Geometry: final body of the model. Coordinates: model frame, mm. Face numbers are marked on the shaded views. A direction names the side the tool comes from. Round coordinates to 2 decimals unless told otherwise and drop trailing zeros. Order: outer loops, then holes, each group sorted by start corner. A loop starts at its lowest first (then second) coordinate and runs counter-clockwise, first axis right, second up. Notation, with made-up numbers: (9.25, -15.5) -> (63.25, -15.5) arc R21 cw to (63.25, 7.5) -> close; hole circle Ø2 at (49, 86). An arc over 180 degrees is marked (long way). Put each result on its own line as item: value.
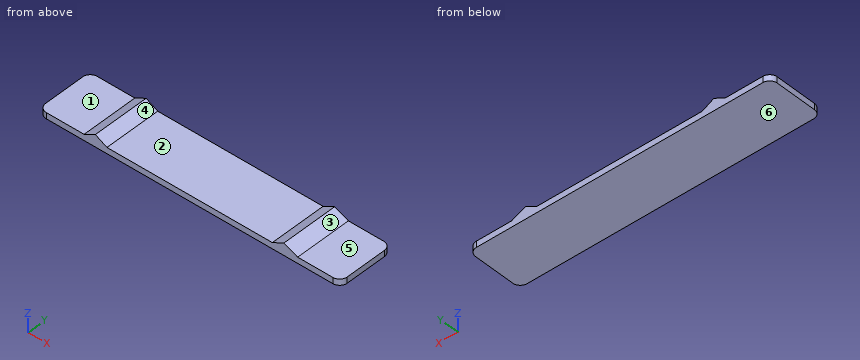
```python
from build123d import *

# Parameters (mm, degrees)
PAD_DEPTH = 7.5
FILLET_R  = 1


with BuildPart() as part:
    # Sketch → Pad (new body)
    with BuildSketch(Plane.XZ):
        Polygon((-20, -0.4), (20, -0.4), (20, 0.4), (14.320997, 0.4), (12.5, 1.2), (10.965424, 0.4), (-10.965424, 0.4), (-12.5, 1.2), (-13.994693, 0.4), (-20, 0.4), align=None)
    extrude(amount=PAD_DEPTH)

    # Fillet
    fillet_edges = [part.edges().sort_by_distance(p)[0] for p in [
        (-20, -7.5, 0),
        (-20, 0, 0),
        (20, 0, 0),
        (20, -7.5, 0),
    ]]
    fillet(fillet_edges, radius=FILLET_R)


solid = part.part
```
1. Draft query along X for the marked faces 1, 2 and 3. Return one class per face: +X half, -X half, draft (parallel to the pull), parting line (faces both ways), or undercut.
Ans:
face 1: draft
face 2: undercut
face 3: +X half
2. Cut plane D-D on y = -0.5. Return loops of the section in (x, z), and give its area (3 significant figures).
Ans:
outline: (-19.87, -0.4) -> (19.87, -0.4) -> (19.87, 0.4) -> (14.32, 0.4) -> (12.5, 1.2) -> (10.97, 0.4) -> (-10.97, 0.4) -> (-12.5, 1.2) -> (-13.99, 0.4) -> (-19.87, 0.4) -> close
area: 34.3 mm²
3. Contact query for a flat-ended pin moving along its axis: P1, Ø1.8, axis at x = -17, y = -5.5, coming from the +Z side. Output: stop coordinate, or through.
Ans:
P1: z = 0.4
4. Cut plane C-C on x = -0.5. Return loops of the section in (y, z).
Ans:
outline: (-7.5, -0.4) -> (0, -0.4) -> (0, 0.4) -> (-7.5, 0.4) -> close
5. Cut plane A-A on z = 0.85. Return loops of the section in (x, y).
Ans:
outline: (-13.15, -7.5) -> (-11.83, -7.5) -> (-11.83, 0) -> (-13.15, 0) -> close; (11.83, -7.5) -> (13.3, -7.5) -> (13.3, 0) -> (11.83, 0) -> close
6. Material intervals for probe 1 along Z at (x, y) = (-0.5, -1.25); probe 2 along X at (y, z) = (-3.5, 0.6); probe 3 along X at (y, z) = (-5, 0.5), sorted ascending.
Ans:
probe 1: -0.4 to 0.4
probe 2: -13.62 to -11.35, 11.35 to 13.87
probe 3: -13.81 to -11.16, 11.16 to 14.09
7. Set-up query: the marked faces 4, 5 and 6. Return all of +Z, -Z, +X, -X, +Y, -Y with unobstructed straight access to the full face (end or side cutting, diameter ignored); none if empty.
Ans:
face 4: +Z, +Y, -Y
face 5: +Z, +X, +Y, -Y
face 6: -Z, +X, -X, +Y, -Y
8. Cut plane B-B on y = -3.25. Return loops of the section in (x, z), and give its area (3 significant figures).
Ans:
outline: (-20, -0.4) -> (20, -0.4) -> (20, 0.4) -> (14.32, 0.4) -> (12.5, 1.2) -> (10.97, 0.4) -> (-10.97, 0.4) -> (-12.5, 1.2) -> (-13.99, 0.4) -> (-20, 0.4) -> close
area: 34.6 mm²
